Design review of the part built by this model. Coordinates are the model's own, in mm. Round coordinates to 2 decimals unless told otherwise and drop trailing zeros. Loops run counter-clockwise (first coordinate to the right, second up) from the corner with the lowest first, then second, coordinate; pieces in that order, holes last. Notation, with made-up numbers: (-8, -10) - (13, -10) arc R35 ccw to (13, 23) - close; hole circle Ø11 at (-15.75, 25.5). An arc over 180 degrees is marked (long way). Use one line per item in the form item = value. Start each with the question number.
(1) We need section C-C, the plane y = 0.9. Write out the cut boundary in (x, z).
(2) We need section A-A, the plane z = -120.5. Write out the cut boundary in (x, y).
(3) Wall thickness on probe 1 along Z at (x, y) = (24.5, 1.4); probe 2 along X at (y, z) = (2.3, 122.5): over which ranges is each line inside the solid? List them lowest first. Write a range as [from, to].
(4) We need section B-B, the plane x = 96. Write out the cut boundary in (y, z).
from build123d import *

# Parameters (mm, degrees)
SKETCH1_W           = 279.4
SKETCH1_H           = 279.4
SKETCH1_W_2         = 117
SKETCH1_H_2         = 30
BOSS_EXTRUDE1_DEPTH = 3


with BuildPart() as part:
    # Sketch1 → Boss-Extrude1 (new body)
    with BuildSketch(Plane(origin=(0, 0, 0), x_dir=(1, 0, 0), z_dir=(0, 1, 0))):
        Rectangle(SKETCH1_W, SKETCH1_H)
        with Locations((-71.2, 119.7)):
            Rectangle(SKETCH1_W_2, SKETCH1_H_2, mode=Mode.SUBTRACT)
        with Locations((71.2, 119.7)):
            Rectangle(SKETCH1_W_2, SKETCH1_H_2, mode=Mode.SUBTRACT)
        with Locations((71.2, -119.7)):
            Rectangle(SKETCH1_W_2, SKETCH1_H_2, mode=Mode.SUBTRACT)
        with Locations((-71.2, -119.7)):
            Rectangle(SKETCH1_W_2, SKETCH1_H_2, mode=Mode.SUBTRACT)
    extrude(amount=BOSS_EXTRUDE1_DEPTH)


solid = part.part
Data:
q1.outline = (-139.7, -139.7) - (139.7, -139.7) - (139.7, 139.7) - (-139.7, 139.7) - close; hole (-129.7, -134.7) - (-12.7, -134.7) - (-12.7, -104.7) - (-129.7, -104.7) - close; hole (-129.7, 104.7) - (-12.7, 104.7) - (-12.7, 134.7) - (-129.7, 134.7) - close; hole (12.7, -134.7) - (129.7, -134.7) - (129.7, -104.7) - (12.7, -104.7) - close; hole (12.7, 104.7) - (129.7, 104.7) - (129.7, 134.7) - (12.7, 134.7) - close
q2.outline = (-139.7, 0) - (-129.7, 0) - (-129.7, 3) - (-139.7, 3) - close; (-12.7, 0) - (12.7, 0) - (12.7, 3) - (-12.7, 3) - close; (129.7, 0) - (139.7, 0) - (139.7, 3) - (129.7, 3) - close
q3.probe_1 = [-139.7, -134.7], [-104.7, 104.7], [134.7, 139.7]
q3.probe_2 = [-139.7, -129.7], [-12.7, 12.7], [129.7, 139.7]
q4.outline = (0, -139.7) - (3, -139.7) - (3, -134.7) - (0, -134.7) - close; (0, -104.7) - (3, -104.7) - (3, 104.7) - (0, 104.7) - close; (0, 134.7) - (3, 134.7) - (3, 139.7) - (0, 139.7) - close
